```python
from build123d import *

# Parameters (mm, degrees)
F0_W     = 100
F0_H     = 150
F1_DEPTH = 10
F7_DEPTH = 177.856339


with BuildPart() as f1:
    # F0 (on Front) → F1 (new body)
    with BuildSketch(Plane.XZ):
        Rectangle(F0_W, F0_H)
    extrude(amount=-F1_DEPTH)

    # F6 (on face) → F7 (cut, through all)
    with BuildSketch(Plane(origin=(-70.710678, -50, 50), x_dir=(0.408248, -0.866025, -0.288675), z_dir=(-0.707107, -0.5, 0.5))):
        Polygon((-16.583499, 6.122708), (-6.122708, -16.583499), (16.583499, -6.122708), (6.122708, 16.583499), align=None)
    extrude(amount=-F7_DEPTH, mode=Mode.SUBTRACT)


solid = f1.part
```
Verification items for the finished model (mm, model axes). A direction names the side the tool comes from. Coordinates: 2 decimals unless noted, no trailing zeros. Write each loop counter-clockwise with the first axis right and the second up, starting at its lowest first coordinate (ties: lowest second). Pieces come first, ordered by that corner, then holes. Notation, with made-up numbers: (1, 27.5) - (6, 27.5) arc R15 cw to (6, 43.5) - close; hole circle Ø6 at (12.25, 81.25). An arc over 180 degrees is marked (long way). One line per question, with ' | ' between items. Start each with the question number.
1. Section check A-A (z = -14). Enter the section's corners in (x, y).
2. Section check B-B (x = 14). Enter the section's corners in (y, z).
3. Section check C-C (y = 3.75). Enter the section's corners in (x, z).
4. Draft check along X on faces 3 (the flat face through (-50, 5, -1)), 4 (the flat face through (50, 5, -1)), 5 (the flat face through (-1, 5, 75)), 6 (the flat face through (8.357, 5.705, -20.318)). Enter one of: released by +X, released by -X, zero draft, split by the parting line, or undercut.
5. Access from +Z, -Z, +X, -X, +Y, -Y to the whole of each face (thin tool, end or side, straight path). Record for faces 1 (the flat face through (-12, 10, 1)), 2 (the flat face through (5.022, 4.885, 10.383)).
6. Gauge pin test, flat end, axial feed: P1, Ø2, axis at x = -16.5, z = -20.5, coming from the -Y side. Record the tip position at first contact, or that the pin passes through.
7. Material ranges on line 1 along Z through (x, y) = (-1.5, 3.25); line 2 along Z through (x, y) = (0, 3.75); line 3 along X through (y, z) = (1.5, 2), recorded low to high.
Computed values:
1) outline: (-50, 0) - (-1.21, 0) - (-8.92, 7.53) - (-5.75, 10) - (-50, 10) - close; (22.23, 0) - (50, 0) - (50, 10) - (35.07, 10) - close
2) outline: (0, -75) - (10, -75) - (10, -24.44) - (0, -20.23) - close; (0, 8.76) - (10, 4.55) - (10, 75) - (0, 75) - close
3) outline: (-50, -75) - (50, -75) - (50, 75) - (-50, 75) - close; hole (-18.24, 20.4) - (-14.27, -10.22) - (28.85, -27.9) - (24.88, 2.72) - close
4) face 3: released by -X | face 4: released by +X | face 5: zero draft | face 6: undercut
5) face 1: +Z, -Z, +X, -X, +Y | face 2: none
6) P1: y = 0
7) line 1: -75 to -15.25, 13.74 to 75 | line 2: -75 to -16.07, 12.92 to 75 | line 3: -50 to -18.75, 22.08 to 50
